```python
from build123d import *

# Parameters (mm, degrees)
F0_W     = 257.175
F0_H     = 206.375
F0_W_2   = 206.375
F0_H_2   = 155.575
F0_R     = 6.35
F1_DEPTH = 6.35
F2_R     = 6.35
F3_DEPTH = 25.4


with BuildPart() as f1:
    # F0 (on Front) → F1 (new body)
    with BuildSketch(Plane.XZ):
        Rectangle(F0_W, F0_H)
        Rectangle(F0_W_2, F0_H_2, mode=Mode.SUBTRACT)
        Rectangle(F0_W_2, F0_H_2)
        with Locations((-77.7875, -52.5145)):
            Circle(F0_R, mode=Mode.SUBTRACT)
        with Locations((-0.0635, -52.5145)):
            Circle(F0_R, mode=Mode.SUBTRACT)
        with Locations((-77.7875, -0.0635)):
            Circle(F0_R, mode=Mode.SUBTRACT)
        with Locations((-0.0635, -0.0635)):
            Circle(F0_R, mode=Mode.SUBTRACT)
        with Locations((77.6605, -52.5145)):
            Circle(F0_R, mode=Mode.SUBTRACT)
        with Locations((77.6605, -0.0635)):
            Circle(F0_R, mode=Mode.SUBTRACT)
        with Locations((-77.7875, 52.3875)):
            Circle(F0_R, mode=Mode.SUBTRACT)
        with Locations((-0.0635, 52.3875)):
            Circle(F0_R, mode=Mode.SUBTRACT)
        with Locations((77.6605, 52.3875)):
            Circle(F0_R, mode=Mode.SUBTRACT)
    extrude(amount=F1_DEPTH)

    # F2 (on face) → F3 (cut)
    with BuildSketch(Plane.XZ.offset(6.35)):
        with Locations((-38.9001, 26.161997)):
            Circle(F2_R)
        with Locations((0.0127, 26.161997)):
            Circle(F2_R)
        with Locations((38.9255, 26.161997)):
            Circle(F2_R)
    extrude(amount=-F3_DEPTH, mode=Mode.SUBTRACT)


solid = f1.part
```
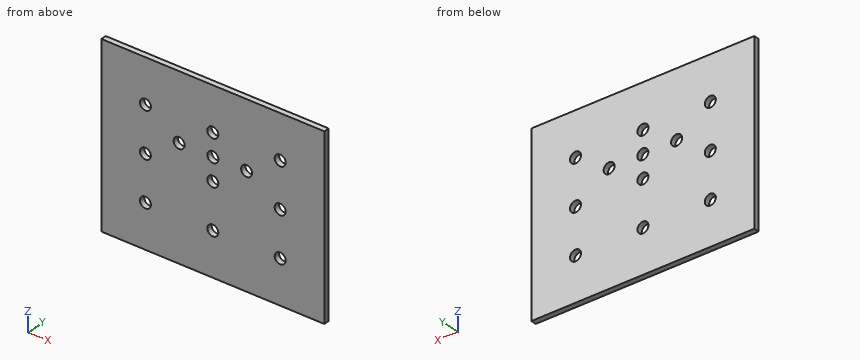
The listing builds one solid part. Answer for the finished solid, in the listing's coordinates (mm). Coordinates: 2 decimals unless noted, no trailing zeros. Write each loop counter-clockwise with the first axis right and the second up, starting at its lowest first coordinate (ties: lowest second). Pieces come first, ordered by that corner, then holes. Notation, with made-up numbers: (-28.5, -11) -> (-21.5, -11) arc R14 ccw to (-21.5, -2) -> close; hole circle Ø2 at (64.25, 75.5). An arc over 180 degrees is marked (long way). Write each question's results on one line, items separated by ' | '. Start each with the question number.
1) A cutting plane is placed at A-A (x = -38.5). Determine the outline of the cut face in (y, z).
2) Straight lines are drawn through the part: probe 1 along X at (y, z) = (-2.5, -0.5); probe 2 along X at (y, z) = (-2.5, 50); probe 3 along Z at (x, y) = (73.5, -4.75). For each, find the intervals that lie inside material, in ascending order.
3) A cutting plane is placed at B-B (y = -2). Count the separate pieces of the cut face and the enclosed holes in it, then the cut area to 3 significant figures.
Values follow:
1) outline: (-6.35, -103.19) -> (0, -103.19) -> (0, 19.82) -> (-6.35, 19.82) -> close; (-6.35, 32.5) -> (0, 32.5) -> (0, 103.19) -> (-6.35, 103.19) -> close
2) probe 1: -128.59 to -84.12, -71.45 to -6.4, 6.27 to 71.33, 84 to 128.59 | probe 2: -128.59 to -83.67, -71.9 to -5.95, 5.82 to 71.78, 83.54 to 128.59 | probe 3: -103.19 to -57.31, -47.72 to -4.86, 4.73 to 47.59, 57.18 to 103.19
3) separate pieces: 1 | enclosed holes: 12 | area: 51,600 mm²
